```python
from build123d import *

# Parameters (mm, degrees)
SKETCH1_W           = 69.0372
SKETCH1_H           = 49.8856
BOSS_EXTRUDE1_DEPTH = 1.778
FILLET1_R           = 0.381
SKETCH2_W           = 59.7662
SKETCH2_H           = 45.1866
CUT_EXTRUDE1_DEPTH  = 0.0254
SKETCH3_R           = 0.4445
BOSS_EXTRUDE2_DEPTH = 0.762
SKETCH5_W           = 19.05
SKETCH5_H           = 40.64
BOSS_EXTRUDE3_DEPTH = 0.381
SKETCH6_W           = 2.571951578
SKETCH6_H           = 11.383775042
SKETCH6_H_2         = 11.011674943
SKETCH6_W_2         = 1.784918448
SKETCH6_H_3         = 1.819764249
SKETCH6_H_4         = 4.247776912
SKETCH6_H_5         = 7.729561266
CUT_EXTRUDE2_DEPTH  = 60.163083243


with BuildPart() as part:
    # Sketch1 → Boss-Extrude1 (new, symmetric)
    with BuildSketch(Plane(origin=(0, 0, 0), x_dir=(1, 0, 0), z_dir=(0, 1, 0))):
        Rectangle(SKETCH1_W, SKETCH1_H)
    extrude(amount=BOSS_EXTRUDE1_DEPTH, both=True)

    # Fillet1
    fillet1_edges = [part.edges().sort_by_distance(p)[0] for p in [
        (34.5186, 0, 24.9428),
        (-34.5186, 0, 24.9428),
        (-34.5186, 0, -24.9428),
        (34.5186, 0, -24.9428),
    ]]
    fillet(fillet1_edges, radius=FILLET1_R)

    # Sketch2 → Cut-Extrude1 (cut)
    with BuildSketch(Plane(origin=(0, 1.778, 0), x_dir=(1, 0, 0), z_dir=(0, 1, 0))):
        with Locations((-3.3655, -0.4445)):
            Rectangle(SKETCH2_W, SKETCH2_H)
    extrude(amount=-CUT_EXTRUDE1_DEPTH, mode=Mode.SUBTRACT)

    # Sketch3 → Boss-Extrude2 (add)
    with BuildSketch(Plane.XZ.offset(1.778)):
        with Locations(Location((-33.9725, 24.4729, 0), (0, 0, 270))):
            Circle(SKETCH3_R)
        with Locations(Location((33.9725, 24.4729, 0), (0, 0, 270))):
            Circle(SKETCH3_R)
        with Locations(Location((33.9725, -24.4729, 0), (0, 0, 270))):
            Circle(SKETCH3_R)
        with Locations(Location((-33.9725, -24.4729, 0), (0, 0, 270))):
            Circle(SKETCH3_R)
    extrude(amount=BOSS_EXTRUDE2_DEPTH)

    # Sketch5 → Boss-Extrude3 (add, symmetric)
    with BuildSketch(Plane(origin=(0, 0, 0), x_dir=(1, 0, 0), z_dir=(0, 1, 0))):
        with Locations((44.0436, 0)):
            Rectangle(SKETCH5_W, SKETCH5_H)
    extrude(amount=BOSS_EXTRUDE3_DEPTH, both=True)

    # Sketch6 → Cut-Extrude2 (cut, through all)
    with BuildSketch(Plane(origin=(0, 0.381, 0), x_dir=(1, 0, 0), z_dir=(0, 1, 0))):
        with Locations((52.282624211, 14.628112479)):
            Rectangle(SKETCH6_W, SKETCH6_H)
        with Locations((52.282624211, -14.814162529)):
            Rectangle(SKETCH6_W, SKETCH6_H_2)
        with Locations((35.411059224, -19.410117875)):
            Rectangle(SKETCH6_W_2, SKETCH6_H_3)
        with Locations((35.411059224, -8.786057404)):
            Rectangle(SKETCH6_W_2, SKETCH6_H_4)
        with Locations((35.411059224, 13.218819714)):
            Rectangle(SKETCH6_W_2, SKETCH6_H_5)
    extrude(amount=-CUT_EXTRUDE2_DEPTH, mode=Mode.SUBTRACT)


solid = part.part
```
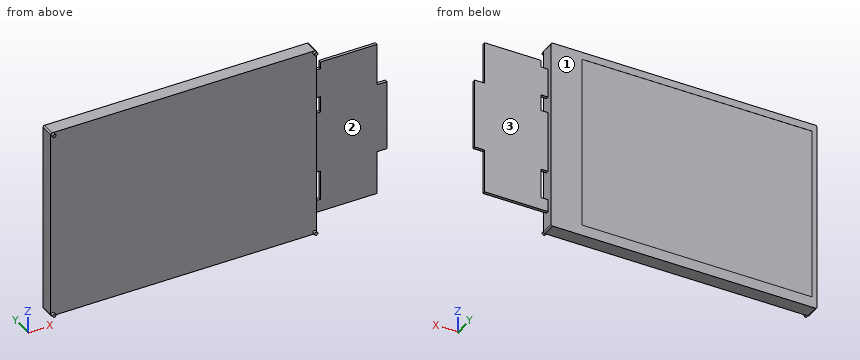
Source: CAD feature listing. Evaluate the final solid. Frame: model axes, mm. Face numbers are marked on the shaded views. A direction names the side the tool comes from. Round coordinates to 2 decimals unless told otherwise and drop trailing zeros. Loops run counter-clockwise (first coordinate to the right, second up) from the corner with the lowest first, then second, coordinate; pieces in that order, holes last. Notation, with made-up numbers: M -32.75,36 L 22.25,36 A21 ccw 22.25,53 Z; hole C 45.5,43 d10. An arc over 180 degrees is marked long. Use a Markdown table: item, result. Add a question column.
1. Contact query for flat-ended pins moving along their axis: pin 1 (0.8 mm diameter, centred on x = 45, y = 0, fed in from -Z); pin 2 (5 mm diameter, centred on x = -19.5, z = -5, fed in from +Y); pin 3 (5.5 mm diameter, centred on x = 46, z = -8.5, fed in from +Y). Output: stop coordinate, or through.
2. Ray query, line 1 along Z through (x, y) = (36, 0); line 2 along X through (y, z) = (1.45, 0.5); line 3 along Y through (x, z) = (0.5, -15). Return the intervals inside material, ascending. Write a range as [from, to].
3. Set-up query: the marked faces 1, 2 and 3. Return all of +Z, -Z, +X, -X, +Y, -Y with unobstructed straight access to the full face (end or side cutting, diameter ignored); none if empty.
4. Cut plane D-D, the plane x = 47. Output: boundary loops of the cut face in (y, z).
Solution:
| question | item | result |
|---|---|---|
| 1 | pin 1 | stops at z = -20.32 |
| 1 | pin 2 | stops at y = 1.75 |
| 1 | pin 3 | stops at y = 0.38 |
| 2 | line 1 | z = [-20.32, -17.08], [-9.35, 6.66], [10.91, 18.5] |
| 2 | line 2 | x = [-34.52, 34.52] |
| 2 | line 3 | y = [-1.78, 1.75] |
| 3 | face 1 | +Z, -Z, +X, -X, +Y |
| 3 | face 2 | +Z, -Z, +X, -Y |
| 3 | face 3 | +Z, -Z, +X, +Y |
| 4 | outline | M -0.38,-20.32 L 0.38,-20.32 L 0.38,20.32 L -0.38,20.32 Z |
